The model under review builds one solid part; all positions refer to its coordinate system, in mm. Face numbers are marked on the shaded views. A direction names the side the tool comes from. Coordinates: 2 decimals unless noted, no trailing zeros. Order: outer loops, then holes, each group sorted by start corner. A loop starts at its lowest first (then second) coordinate and runs counter-clockwise, first axis right, second up.
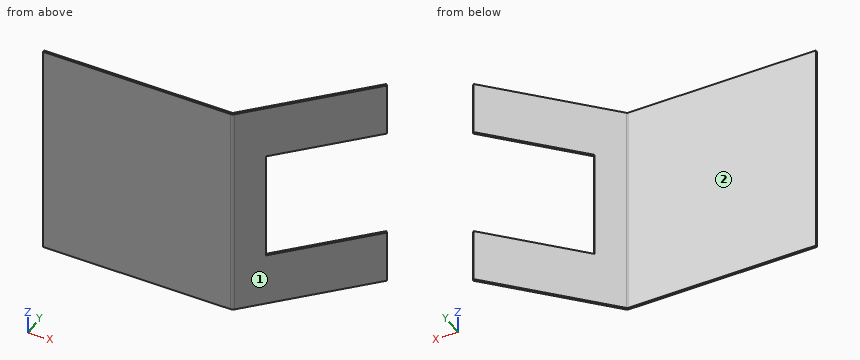
Autodesk Inventor part; units mm, degrees
ref_plane "YZ Plane" through (0, 0, 0) normal (1, 0, 0) x (0, 1, 0)
ref_plane "XZ Plane" through (0, 0, 0) normal (0, 1, 0) x (-1, 0, 0)
ref_plane "XY Plane" through (0, 0, 0) normal (0, 0, 1) x (1, 0, 0)
sketch "Sketch1" plane through (0, 0, 0) normal (0, 1, 0) x (-1, 0, 0)
  line L0 (0, 0) -> (169.946, 0)
  line L1 (169.946, 0) -> (169.946, -197)
  line L2 (169.946, -197) -> (0, -197)
  line L3 (0, -197) -> (0, 0)
  dimension "d0" = 197
  dimension "d1" = 169.946
extrude "Plate1" add sketch "Sketch1" along normal blind 2
sketch "Sketch2" plane through (-1.4142, 1.4142, -197) normal (0.7071068, -0.7071068, 0) x (0.7071068, 0.7071068, 0)
  line L0 (0, 197) -> (0, 0)
  line L1 (0, 0) -> (127.842, 0)
  line L2 (127.842, 0) -> (127.842, 197)
  line L3 (127.842, 197) -> (0, 197)
edge flange "Flange1" height 127.842 angle 45 thickness 2 bend radius 2 thickness toward (0.7071068, -0.7071068, 0) relief tear relief width 2 relief depth 1 edges at (0, 2, -98.5) wall of the first edge with corners at (-1.4142, 1.4142, 0) (-1.4142, 1.4142, -197) (88.9837, 91.8122, -197) (88.9837, 91.8122, 0)
bend "Bend1"
corner "Corner1"
sketch "Sketch3" plane through (90.3979, 90.3979, 0) normal (0.7071068, -0.7071068, 0) x (-0.7071068, -0.7071068, 0)
  line L0 (0, 48.5) -> (100, 48.5)
  line L1 (100, 48.5) -> (100, 148.5)
  line L2 (100, 148.5) -> (0, 148.5)
  line L3 (0, 148.5) -> (0, 48.5)
  line L4 (0, 197) -> (126.1851, 197)
  line L5 (0, 0) -> (0, 197)
  point P0 (127.842, 0)
  point P1 (63.0926, 197)
  dimension "d13" = 100
  dimension "d14" = 100
  dimension "d15" = 48.5
extrude "Cut1" cut sketch "Sketch3" against normal blind 2
equation "\"d14\" = d13"
equation "\"d16\" = Thickness"
equation "\"d2\" = Thickness"
equation "\"d3\" = BendReliefWidth"
equation "\"d4\" = BendReliefDepth"
equation "\"d5\" = MinimumRemnant"
equation "\"d6\" = TransitionRadius"
equation "\"d9\" = BendRadius"
equation "\"d10\" = CornerReliefSize"
equation "\"d11\" = GapSize"
equation "\"d12\" = JacobiRadiusSize"
equation "\"BendRadius\" = Thickness"
equation "\"BendReliefWidth\" = Thickness"
equation "\"BendReliefDepth\" = 0.5 * Thickness"
equation "\"CornerReliefSize\" = 4 * Thickness"
equation "\"MinimumRemnant\" = 2 * Thickness"
equation "\"TransitionRadius\" = BendRadius"
equation "\"JacobiRadiusSize\" = BendRadius"
equation "\"GapSize\" = Thickness"
properties part number "LzC-FrontPLateRS3" material "Steel"
(1) Wall thickness on probe 1 along Y at (x, z) = (-89, -128); probe 2 along X at (y, z) = (71, -186.5); probe 3 along X at (y, z) = (60.5, -33): over which ranges is each line inside the solid? List them lowest first.
A:
probe 1: y = 0 to 2
probe 2: x = 68.17 to 71
probe 3: x = 57.67 to 60.5
(2) For pin 1 Ø2 at (y, z) = (43.5, -24) entering from +X; pin 2 Ø5 at (y, z) = (44, -21.5) entering from -X; pin 3 Ø2 at (y, z) = (67.5, -166.5) entering from +X; pin 4 Ø2 at (x, z) = (-135.5, -77) entering from -Y, all flat-tipped, find the tip position at first contact; note any pin that passes through.
A:
pin 1: stops at x = 44.5
pin 2: stops at x = 38.67
pin 3: stops at x = 68.5
pin 4: stops at y = 0
(3) Machinability: for the marked faces 1 and 2, which of the approach directions +Z, -Z, +X, -X, +Y, -Y give a long, thin tool a straight path to every point of the face, cutting with its end or side? Answer none if there is none.
A:
face 1: +Z, -Z, +X, -Y
face 2: +Z, -Z, -X, +Y
(4) We need section C-C, the plane z = -92. Write out the cut boundary in (x, y).
A:
outline: (-169.95, 0) - (-1.66, 0) arc R4 ccw to (1.17, 1.17) - (19.69, 19.69) - (18.27, 21.1) - (-0.24, 2.59) arc R2 cw to (-1.66, 2) - (-169.95, 2) - close
(5) We need section D-D, the plane x = -17.5. Write out the cut boundary in (y, z).
A:
outline: (0, -197) - (2, -197) - (2, 0) - (0, 0) - close
(6) We need section A-A, the plane x = 30. Write out the cut boundary in (y, z), and give its area (3 significant figures).
A:
outline: (30, -197) - (32.83, -197) - (32.83, -148.5) - (30, -148.5) - close; (30, -48.5) - (32.83, -48.5) - (32.83, 0) - (30, 0) - close
area: 274 mm2
(7) We need section B-B, the plane y = 72. Write out the cut boundary in (x, z).
A:
outline: (69.17, -197) - (72, -197) - (72, -148.5) - (69.17, -148.5) - close; (69.17, -48.5) - (72, -48.5) - (72, 0) - (69.17, 0) - close
